from build123d import *

# Parameters (mm, degrees)
SKETCH_1_W          = 11
SKETCH_1_H          = 20
EXTRUDE_1_DEPTH     = 1
SKETCH_2_R          = 1.15
CUT_EXTRUDE_1_DEPTH = 12.586630226
FILLET_1_R          = 2


with BuildPart() as part:
    # 草图1 → 凸台-拉伸1 (new, symmetric)
    with BuildSketch(Plane.XY):
        Rectangle(SKETCH_1_W, SKETCH_1_H)
    extrude(amount=EXTRUDE_1_DEPTH, both=True)

    # 草图2 → 切除-拉伸1 (cut, through all)
    with BuildSketch(Plane.XY.offset(1)):
        with Locations((-2.5, 8)):
            Circle(SKETCH_2_R)
        with Locations((2.5, 8)):
            Circle(SKETCH_2_R)
        with Locations((-2.5, -8)):
            Circle(SKETCH_2_R)
        with Locations((2.5, -8)):
            Circle(SKETCH_2_R)
    extrude(amount=-CUT_EXTRUDE_1_DEPTH, mode=Mode.SUBTRACT)

    # 圆角1
    fillet_1_edges = [part.edges().sort_by_distance(p)[0] for p in [
        (5.5, -10, 0),
        (-5.5, -10, 0),
        (-5.5, 10, 0),
        (5.5, 10, 0),
    ]]
    fillet(fillet_1_edges, radius=FILLET_1_R)


solid = part.part
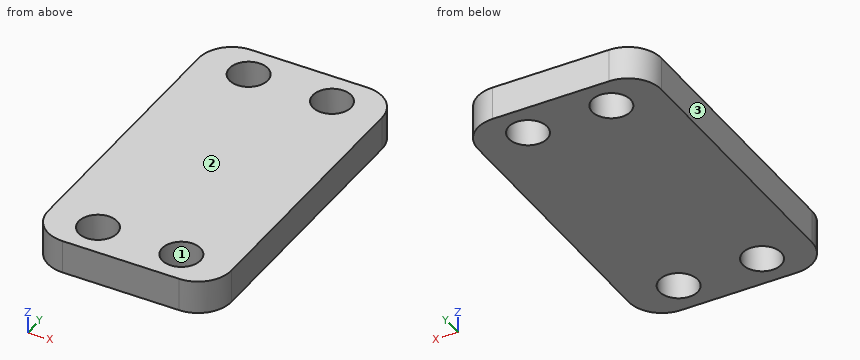
Read the model definition and answer for the solid it produces. Units are mm, in the model's axes. Face numbers are marked on the shaded views. Round coordinates to 2 decimals unless told otherwise and drop trailing zeros. Write each loop counter-clockwise with the first axis right and the second up, starting at its lowest first coordinate (ties: lowest second). Pieces come first, ordered by that corner, then holes.
1. The part is cut by section B-B, the plane z = -0.55. Determine the outline of the cut face in (x, y).
2. Straight lines are drawn through the part: L1, parallel to Y at x = 2.5, z = 0.2; L2, parallel to X at y = 7.25, z = 0.65; L3, parallel to Y at x = 3.25, z = 0.8. For each, find the intervals that lie inside material, in ascending order.
3. The part is cut by section C-C, the plane x = -4.5. Determine the outline of the cut face in (y, z).
4. Given pin 1 Ø2 at (x, y) = (2.5, -8) entering from -Z, flat-ended and moving along its own axis, determine where the tip first touches the part or whether it passes through.
5. Determine the mould class of the marked faces 1, 2 and 3 for opening direction X: pulls with the +X half, pulls with the -X half, needs draft (parallel to the pull), parting line crosses it, or undercut.
6. The part is cut by section A-A, the plane x = -2.5. Determine the outline of the cut face in (y, z).
Values:
1. outline: (-5.5, -8) arc R2 ccw to (-3.5, -10) - (3.5, -10) arc R2 ccw to (5.5, -8) - (5.5, 8) arc R2 ccw to (3.5, 10) - (-3.5, 10) arc R2 ccw to (-5.5, 8) - close; hole circle Ø2.3 at (-2.5, -8); hole circle Ø2.3 at (-2.5, 8); hole circle Ø2.3 at (2.5, -8); hole circle Ø2.3 at (2.5, 8)
2. L1: y = -10 to -9.15, -6.85 to 6.85, 9.15 to 10
2. L2: x = -5.5 to -3.37, -1.63 to 1.63, 3.37 to 5.5
2. L3: y = -10 to -8.87, -7.13 to 7.13, 8.87 to 10
3. outline: (-9.73, -1) - (9.73, -1) - (9.73, 1) - (-9.73, 1) - close
4. pin 1: passes through
5. face 1: undercut
5. face 2: needs draft
5. face 3: pulls with the -X half
6. outline: (-10, -1) - (-9.15, -1) - (-9.15, 1) - (-10, 1) - close; (-6.85, -1) - (6.85, -1) - (6.85, 1) - (-6.85, 1) - close; (9.15, -1) - (10, -1) - (10, 1) - (9.15, 1) - close
